Here's how the part is built. I have some questions about the finished solid (model axes, mm). A direction names the side the tool comes from. Coordinates: 2 decimals unless noted, no trailing zeros. Order: outer loops, then holes, each group sorted by start corner. A loop starts at its lowest first (then second) coordinate and runs counter-clockwise, first axis right, second up. Notation, with made-up numbers: (32, -1.75) - (40, -1.75) arc R19 ccw to (40, 8.25) - close; hole circle Ø7 at (84, 19.5). An arc over 180 degrees is marked (long way). Answer as CSV lines item,"result". Start each with the question number.
Item 1: Imagine slicing it at B-B on z = 4. List the corners of the cut face in (x, y) for me.
Item 2: Imagine slicing it at C-C on y = -3.75. Count the separate pieces of the cut face and the enclosed holes in it, and give its area (3 significant figures).
Item 3: Imagine slicing it at D-D on x = 16. List the corners of the cut face in (y, z) for me, and give its area (3 significant figures).
Item 4: We'd pull the mould along Z, two halves only. Please class faces 1 (the face through (-6, 0, 1)), 2 (the face through (20.661, -2.535, 24.843)), 3 (the face through (20.42, -2.54, -24.98)), 4 (the face through (6.461, -2.535, -11.975)): pulls with the +Z half, pulls with the -Z half, needs draft (parallel to the pull), parting line crosses it, or undercut.
Item 5: On a 3-axis mill with a long thin cutter (end or side, diameter ignored), from which of +Z, -Z, +X, -X, +Y, -Y can I reach the whole of each face in a straight line? I mean faces 5 (the face through (23.025, -2.535, 4.966)), 6 (the face through (-38, -3, 15.774)). Say none if no direction works.
Item 6: I need wall thicknesses on line 1 (X direction, y = -3.05, z = 13); line 2 (X direction, y = -1.55, z = 5.5); line 3 (Z direction, x = -21.5, y = -1.85). Which ranges of each line are inside material? Lowest first, please.
Item 7: Imagine slicing it at A-A on x = -17. List the corners of the cut face in (y, z) for me.
Item 8: I'm going to push flat-ended pins straight in: pin 1 (2.5 mm diameter, centred on x = -35.75, z = 22.77, fed in from +Y); pin 2 (1.5 mm diameter, centred on y = -3.5, z = -5.5, fed in from -X). Where does each tip first touch, or does it pass through?
from build123d import *

# Parameters (mm, degrees)
SKETCH1_R           = 2.25
SKETCH1_R_2         = 11.5
BOSS_EXTRUDE1_DEPTH = 5


with BuildPart() as part:
    # Sketch1 → Boss-Extrude1 (new body)
    with BuildSketch(Plane.XZ.offset(5)):
        Polygon((-35.75064294, 15.774393454), (-35.75064294, -15.774393454), (-40.75064294, -15.774393454), (-40.75064294, -39.112565995), (-10.75064294, -39.112565995), (11.828174009, -29.823562546), (29.24935706, -20), (29.24935706, 20), (11.828174009, 29.823562546), (-10.75064294, 39.112565995), (-40.75064294, 39.112565995), (-40.75064294, 15.774393454), align=None)
        with Locations((-30.75064294, -22.774393454)):
            Circle(SKETCH1_R, mode=Mode.SUBTRACT)
        with Locations((25.272832985, -3.329685731)):
            Circle(SKETCH1_R, mode=Mode.SUBTRACT)
        with Locations((8.246602308, -10.606066633)):
            Circle(SKETCH1_R, mode=Mode.SUBTRACT)
        with Locations((25.272832985, 4.867552465)):
            Circle(SKETCH1_R, mode=Mode.SUBTRACT)
        with Locations((-30.75064294, -32.112565995)):
            Circle(SKETCH1_R, mode=Mode.SUBTRACT)
        with Locations((-17.003397692, 11.878643261)):
            Circle(SKETCH1_R_2, mode=Mode.SUBTRACT)
        with Locations((8.246602308, 12.143933367)):
            Circle(SKETCH1_R, mode=Mode.SUBTRACT)
        with Locations((-35.75064294, 22.774393454)):
            Circle(SKETCH1_R, mode=Mode.SUBTRACT)
        with Locations((-35.75064294, 32.112565995)):
            Circle(SKETCH1_R, mode=Mode.SUBTRACT)
    extrude(amount=-BOSS_EXTRUDE1_DEPTH)


solid = part.part
Responses:
1,outline,"(-35.75, -5) - (-25.38, -5) - (-25.38, 0) - (-35.75, 0) - close; (-8.63, -5) - (23.2, -5) - (23.2, 0) - (-8.63, 0) - close; (27.35, -5) - (29.25, -5) - (29.25, 0) - (27.35, 0) - close"
2,separate pieces,"1"
2,enclosed holes,"9"
2,area,"4,070 mm^2"
3,outline,"(-5, -27.47) - (0, -27.47) - (0, 27.47) - (-5, 27.47) - close"
3,area,"275 mm^2"
4,face 1,"needs draft"
4,face 2,"pulls with the +Z half"
4,face 3,"pulls with the -Z half"
4,face 4,"undercut"
5,face 5,"+Y, -Y"
5,face 6,"-X, +Y, -Y"
6,line 1,"x = -35.75 to -28.45, -5.56 to 6.17, 10.33 to 29.25"
6,line 2,"x = -35.75 to -26.57, -7.43 to 23.11, 27.43 to 29.25"
6,line 3,"z = -39.11 to 1.29, 22.46 to 39.11"
7,outline,"(-5, -39.11) - (0, -39.11) - (0, 0.38) - (-5, 0.38) - close; (-5, 23.38) - (0, 23.38) - (0, 39.11) - (-5, 39.11) - close"
8,pin 1,"passes through"
8,pin 2,"stops at x = -35.75"
